```python
from build123d import *

# Parameters (mm, degrees)
SKETCH1_R                               = 8
BOSS_EXTRUDE1_DEPTH                     = 10
SKETCH2_R                               = 12.5
CUT_EXTRUDE1_DEPTH                      = 10
SKETCH3_R                               = 3.5
CUT_EXTRUDE2_DEPTH                      = 21
SKETCH4_R                               = 6
CUT_EXTRUDE3_DEPTH                      = 6
CUT_EXTRUDE4_DEPTH                      = 4
FILLET1_R                               = 2
TAP_DRILL_FOR_M10X1_25_TAP1_D           = 8.8
TAP_DRILL_FOR_M10X1_25_TAP1_DEPTH       = 13
TAP_DRILL_FOR_M10X1_25_TAP1_CSINK_D     = 8.85
TAP_DRILL_FOR_M10X1_25_TAP1_CSINK_ANGLE = 90
TAP_DRILL_FOR_M10X1_25_TAP1_TIP         = 2.643786724
FILLET1_OF_MIRROR4_R                    = 2


with BuildPart() as part:
    # Sketch1 → Boss-Extrude1 (new body, symmetric)
    with BuildSketch(Plane.XY):
        with BuildLine():
            Line((-46, 0), (-46, -125))
            Line((-46, -125), (46, -125))
            Line((46, -125), (46, 0))
            ThreePointArc((46, 0), (0, 46), (-46, 0))
        make_face()
        Circle(SKETCH1_R, mode=Mode.SUBTRACT)
    extrude(amount=BOSS_EXTRUDE1_DEPTH, both=True)

    # Sketch2 → Cut-Extrude1 (cut)
    with BuildSketch(Plane.XY.offset(10)):
        Circle(SKETCH2_R)
    extrude(amount=-CUT_EXTRUDE1_DEPTH, mode=Mode.SUBTRACT)

    # Sketch3 → Cut-Extrude2 (cut, through all)
    with BuildSketch(Plane.XY.offset(10)):
        with Locations((0, 39)):
            Circle(SKETCH3_R)
        with Locations((33.774990748, 19.5)):
            Circle(SKETCH3_R)
        with Locations((33.774990748, -19.5)):
            Circle(SKETCH3_R)
        with Locations((0, -39)):
            Circle(SKETCH3_R)
        with Locations((-33.774990748, -19.5)):
            Circle(SKETCH3_R)
        with Locations((-33.774990748, 19.5)):
            Circle(SKETCH3_R)
    extrude(amount=-CUT_EXTRUDE2_DEPTH, mode=Mode.SUBTRACT)

    # Sketch4 → Cut-Extrude3 (cut)
    with BuildSketch(Plane(origin=(0, 0, -10), x_dir=(-1, 0, 0), z_dir=(0, 0, -1))):
        with Locations((0, 39)):
            Circle(SKETCH4_R)
        with Locations((33.774990748, 19.5)):
            Circle(SKETCH4_R)
        with Locations((33.774990748, -19.5)):
            Circle(SKETCH4_R)
        with Locations((0, -39)):
            Circle(SKETCH4_R)
        with Locations((-33.774990748, -19.5)):
            Circle(SKETCH4_R)
        with Locations((-33.774990748, 19.5)):
            Circle(SKETCH4_R)
    extrude(amount=-CUT_EXTRUDE3_DEPTH, mode=Mode.SUBTRACT)

    # Sketch5 → Cut-Extrude4 (cut)
    with BuildSketch(Plane.XY.offset(10)):
        with BuildLine():
            Line((-34, -50.793700397), (-34, -107))
            ThreePointArc((-34, -107), (-32.242640687, -111.242640687), (-28, -113))
            Line((-28, -113), (28, -113))
            ThreePointArc((28, -113), (32.242640687, -111.242640687), (34, -107))
            Line((34, -107), (34, -50.793700397))
            ThreePointArc((34, -50.793700397), (31.051285766, -45.627497229), (25.103448276, -45.539179666))
            ThreePointArc((25.103448276, -45.539179666), (0, -52), (-25.103448276, -45.539179666))
            ThreePointArc((-25.103448276, -45.539179666), (-31.051285766, -45.627497229), (-34, -50.793700397))
        make_face()
    cut_extrude4 = extrude(amount=-CUT_EXTRUDE4_DEPTH, mode=Mode.SUBTRACT)

    # Fillet1
    fillet1_edges = [part.edges().sort_by_distance(p)[0] for p in [
        (32.242640687, -111.242640687, 10),
        (34, -78.896850198, 10),
        (31.051285766, -45.627497229, 10),
        (0, -52, 10),
        (-31.051285766, -45.627497229, 10),
        (-34, -78.896850198, 10),
        (-32.242640687, -111.242640687, 10),
        (0, -113, 10),
    ]]
    fillet(fillet1_edges, radius=FILLET1_R)

    # Tap Drill for M10x1.25 Tap1
    with Locations(Plane(origin=(0, -125, 0), x_dir=(-1, 0, 0), z_dir=(0, -1, 0))):
        with Locations((30, 0), (-30, 0)):
            CounterSinkHole(TAP_DRILL_FOR_M10X1_25_TAP1_D / 2, TAP_DRILL_FOR_M10X1_25_TAP1_CSINK_D / 2, depth=TAP_DRILL_FOR_M10X1_25_TAP1_DEPTH, counter_sink_angle=TAP_DRILL_FOR_M10X1_25_TAP1_CSINK_ANGLE)
            with Locations((0, 0, -(TAP_DRILL_FOR_M10X1_25_TAP1_DEPTH + TAP_DRILL_FOR_M10X1_25_TAP1_TIP / 2))):  # 118° drill point
                Cone(0, TAP_DRILL_FOR_M10X1_25_TAP1_D / 2, TAP_DRILL_FOR_M10X1_25_TAP1_TIP, mode=Mode.SUBTRACT)

    # Mirror4: Cut-Extrude4 across plane
    add(cut_extrude4.mirror(Plane.XY), mode=Mode.SUBTRACT)

    # Fillet1 of Mirror4
    fillet1_of_mirror4_edges = [part.edges().sort_by_distance(p)[0] for p in [
        (32.242640687, -111.242640687, -10),
        (34, -78.896850198, -10),
        (31.051285766, -45.627497229, -10),
        (0, -52, -10),
        (-31.051285766, -45.627497229, -10),
        (-34, -78.896850198, -10),
        (-32.242640687, -111.242640687, -10),
        (0, -113, -10),
    ]]
    fillet(fillet1_of_mirror4_edges, radius=FILLET1_OF_MIRROR4_R)


solid = part.part
```
Model file for the job. Use its own axes, mm. A direction names the side the tool comes from. Give positions to 0.01 mm unless a question says otherwise; leave off trailing zeros. Order: outer loops, then holes, each group sorted by start corner. A loop starts at its lowest first (then second) coordinate and runs counter-clockwise, first axis right, second up.
1) 3-axis set-ups, long thin cutter, end or side, ignore diameter. For faces 4 (the cylindrical face through (30.55, -14.44, -7.04)), 5 (the flat face through (-0.2, -8.2, 0)), 6 (the cylindrical face through (31.2, -17.13, 3.1)): which of +Z, -Z, +X, -X, +Y, -Y reach the whole face in a straight line?
2) Mould opens along Z. For faces 1 (the flat face through (-3, -42, -4)), 2 (the conical face through (-30.729, -109.815, -0.23)), 3 (the cylindrical face through (-30.976, -45.584, -7.014)) say: +Z half, -Z half, draft (parallel to the pull), parting line (faces both ways), or undercut.
3) Saw through at D-D, the plane y = 39. Write the cut outline in (x, z), then the cut area to 3 significant figures.
4) Saw through at A-A, the plane y = -19.5. Write the cut outline in (x, z) (3 decimals).
5) Wall check: probe 1 along Y at (x, z) = (0, -5.3); probe 2 along X at (y, z) = (-16.5, 8.25); probe 3 along X at (y, z) = (-16.5, -7). Give the ranges that are in metal, low to high.
6) Saw through at C-C, the plane y = -64.5. Write the cut outline in (x, z).
7) Pin check, flat tips, straight feed: pin 1 (0.6 mm diameter, centred on x = -7, z = -6.5, fed in from +Y); pin 2 (5.5 mm diameter, centred on x = -33.77, y = -19.5, fed in from +Z); pin 3 (5.5 mm diameter, centred on x = -30, z = 0, fed in from +Y); pin 4 (0.6 mm diameter, centred on x = 5.5, z = 7, fed in from +Y). Stop position of each tip, or through.
8) Saw through at B-B, the plane y = 4. Write the cut outline in (x, z), then the cut area to 3 significant figures.
Computed:
1. face 4: -Z
1. face 5: +Z
1. face 6: +Z, -Z
2. face 1: -Z half
2. face 2: undercut
2. face 3: draft
3. outline: (-24.39, -10) - (-6, -10) - (-6, -4) - (-3.5, -4) - (-3.5, 10) - (-24.39, 10) - close; (3.5, -4) - (6, -4) - (6, -10) - (24.39, -10) - (24.39, 10) - (3.5, 10) - close
3. area: 806 mm2
4. outline: (-46, -10) - (-39.775, -10) - (-39.775, -4) - (-37.275, -4) - (-37.275, 10) - (-46, 10) - close; (-30.275, -4) - (-27.775, -4) - (-27.775, -10) - (27.775, -10) - (27.775, -4) - (30.275, -4) - (30.275, 10) - (-30.275, 10) - close; (37.275, -4) - (39.775, -4) - (39.775, -10) - (46, -10) - (46, 10) - (37.275, 10) - close
5. probe 1: y = -125 to -45, -33 to -8, 8 to 33, 45 to 46
5. probe 2: x = -46 to -35.58, -31.97 to 31.97, 35.58 to 46
5. probe 3: x = -46 to -38.97, -28.58 to 28.58, 38.97 to 46
6. outline: (-46, -10) - (-36, -10) arc R2 ccw to (-34, -8) - (-34, -6) - (34, -6) - (34, -8) arc R2 ccw to (36, -10) - (46, -10) - (46, 10) - (36, 10) arc R2 ccw to (34, 8) - (34, 6) - (-34, 6) - (-34, 8) arc R2 ccw to (-36, 10) - (-46, 10) - close
7. pin 1: stops at y = 45.51
7. pin 2: passes through
7. pin 3: stops at y = 37.06
7. pin 4: stops at y = 45.71
8. outline: (-45.83, -10) - (-6.93, -10) - (-6.93, 0) - (-11.84, 0) - (-11.84, 10) - (-45.83, 10) - close; (6.93, -10) - (45.83, -10) - (45.83, 10) - (11.84, 10) - (11.84, 0) - (6.93, 0) - close
8. area: 1,460 mm2
